Design review of the part built by this model. Coordinates are the model's own, in mm. Face numbers are marked on the shaded views. A direction names the side the tool comes from. Give positions to 0.01 mm unless a question says otherwise; leave off trailing zeros. Loops run counter-clockwise (first coordinate to the right, second up) from the corner with the lowest first, then second, coordinate; pieces in that order, holes last. Notation, with made-up numbers: (23, 75.25) -> (39, 75.25) arc R18 ccw to (39, 90.25) -> close; hole circle Ø9 at (47, -38). An arc over 180 degrees is marked (long way). Answer in a Markdown table with one row per item. Add a question column.
(1) For line 1 (Z direction, x = 7.5, y = -46.5); line 2 (Z direction, x = 11.5, y = 6.5); line 3 (Y direction, x = 7.5, z = -3.5), list the stretches that pass through material, from the lowest coordinate up.
(2) For pin 1 (6.5 mm diameter, centred on x = 7.5, z = 15, fed in from +Y); pin 2 (6 mm diameter, centred on x = 11, y = -3.5, fed in from -Z); pin 3 (5 mm diameter, centred on x = 7.5, y = 8.48, fed in from +Z); pin 4 (3 mm diameter, centred on x = 7.5, z = -15, fed in from +Y), all flat-tipped, find the tip position at first contact; note any pin that passes through.
(3) Consider section D-D on x = 3.25. Write out the cut boundary in (y, z).
(4) Draft analysis for pull direction Y (two halves, no side actions). For the marked faces 4, 5 and 6, state which applies: +Y half, -Y half, draft (parallel to the pull), parting line (faces both ways), or undercut.
(5) Consider section A-A on y = 0. Write out the cut boundary in (x, z).
(6) For the marked faces 1, 2 and 3, list the 3-axis set-ups (+Z, -Z, +X, -X, +Y, -Y) from which the entire face can be reached by the end or side of a thin tool; tool diameter is ignored.
(7) Consider section C-C on z = -15. Write out the cut boundary in (x, y).
(8) Consider section B-B on x = 7.5. Write out the cut boundary in (y, z).
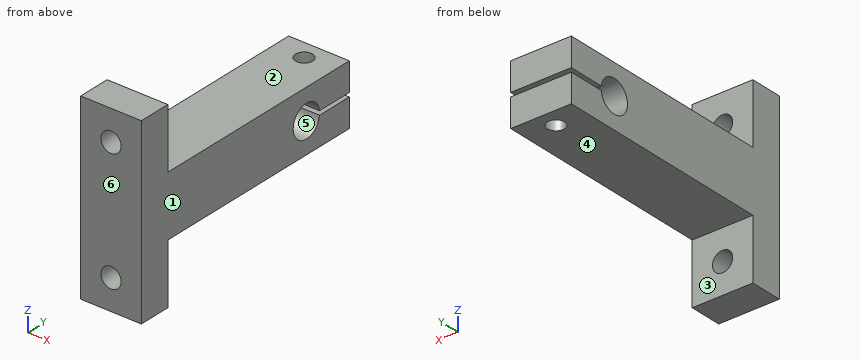
Autodesk Inventor part; units mm, degrees
ref_plane "YZ Plane" through (0, 0, 0) normal (1, 0, 0) x (0, 1, 0)
ref_plane "XZ Plane" through (0, 0, 0) normal (0, 1, 0) x (-1, 0, 0)
ref_plane "XY Plane" through (0, 0, 0) normal (0, 0, 1) x (1, 0, 0)
sketch "Sketch1" plane through (0, 0, 0) normal (1, 0, 0) x (0, 1, 0)
  line L0 (-50, 22.5) -> (-50, -22.5)
  line L1 (-50, -22.5) -> (-42, -22.5)
  line L2 (-42, -22.5) -> (-42, -7.5)
  line L3 (-42, -7.5) -> (13, -7.5)
  line L4 (13, -7.5) -> (13, -0.5)
  line L5 (-50, 22.5) -> (-42, 22.5)
  line L6 (-42, 22.5) -> (-42, 7.5)
  line L7 (-42, 7.5) -> (13, 7.5)
  line L8 (13, 7.5) -> (13, 0.5)
  circle A0 centre (0, 0) radius 4
  line L9 (13, 0.5) -> (0, 0.5)
  line L10 (0, 0.5) -> (0, -0.5)
  line L11 (0, -0.5) -> (13, -0.5)
  line L12 (0, 0) -> (-35.797, 0) construction
  dimension "d0" = 8
  dimension "d1" = 1
  dimension "d2" = 7
  dimension "d3" = 15
  dimension "d5" = 55
  dimension "d6" = 8
  dimension "d11" = 50
extrude "Extrusion1" add sketch "Sketch1" along normal blind 15 contours L5 L6 L7 L8 L9 A0 L11 L4 L3 L2 L1 L0 | L9 L10 L11 A0 picked at (-1.3236, -0.1605)
extrude "Extrusion2" cut sketch "Sketch1" along normal through all contours L9 L10 L11 A0 | A0 L11 L10 L9
sketch "Sketch2" plane through (0, -42, 22.5) normal (0, 1, 0) x (1, 0, 0)
  circle A0 centre (7.5, 7.5) radius 2.5
  circle A1 centre (7.5, 37.5) radius 2.5
  line L0 (0, 45) -> (0, 30)
  line L1 (0, 15) -> (0, 0)
  line L2 (0, 45) -> (0, 30)
  line L3 (0, 30) -> (15, 30)
  line L4 (15, 45) -> (15, 30)
  line L5 (0, 45) -> (15, 45)
  line L6 (0, 15) -> (0, 0)
  line L7 (0, 0) -> (15, 0)
  line L8 (15, 15) -> (15, 0)
  line L9 (0, 15) -> (15, 15)
  line L10 (7.5, 7.5) -> (0, 7.5)
  line L11 (0, 0) -> (0, 45)
  line L12 (7.5, 37.5) -> (15, 37.5)
  line L13 (15, 0) -> (15, 45)
  line L14 (7.5, 37.5) -> (0, 37.5)
  line L15 (7.5, 37.5) -> (7.5, 30)
  line L16 (7.5, 37.5) -> (7.5, 45)
  line L17 (0, 45) -> (15, 45)
  line L18 (7.5, 7.5) -> (15, 7.5)
  line L19 (7.5, 7.5) -> (7.5, 15)
  line L20 (0, 15) -> (15, 15)
  line L21 (7.5, 7.5) -> (7.5, 0)
  line L22 (0, 0) -> (15, 0)
  point P0 (0, 22.5)
  dimension "d12" = 5
extrude "Extrusion3" cut sketch "Sketch2" against normal through all contours L18 L19 A0 | A0 L21 L18 | L19 L10 A0 | A0 L10 L21 | L15 L12 A1 | A1 L14 L15 | L12 L16 A1 | A1 L16 L14
sketch "Sketch3" plane through (0, -42, 7.5) normal (0, 0, 1) x (1, 0, 0)
  circle A0 centre (7.5, 50.4843) radius 2.125
  line L0 (7.5, 50.4843) -> (0, 50.4843) construction
  line L1 (7.5, 50.4843) -> (15, 50.4843) construction
  line L2 (0, 55) -> (0, 0)
  line L3 (0, 55) -> (15, 55)
  line L4 (15, 45.9686) -> (15, 55)
  line L5 (15, 55) -> (15, 0)
  line L6 (7.5, 50.4843) -> (15, 55) construction
  line L7 (15, 45.9686) -> (15, 38)
  line L8 (15, 45.9686) -> (7.5, 50.4843) construction
  point P0 (0, 42)
  point P1 (15, 42)
  dimension "d15" = 4.25
extrude "Extrusion4" cut sketch "Sketch3" against normal through all
properties part number "XRodClamp"
Values follow:
| question | item | result |
|---|---|---|
| 1 | line 1 | -22.5 to -17.5, -12.5 to 12.5, 17.5 to 22.5 |
| 1 | line 2 | -7.5 to -0.5, 0.5 to 7.5 |
| 1 | line 3 | -50 to -1.94, 1.94 to 6.36, 10.61 to 13 |
| 2 | pin 1 | y = -42 |
| 2 | pin 2 | z = -7.5 |
| 2 | pin 3 | z = 7.5 |
| 2 | pin 4 | through |
| 3 | outline | (-50, -22.5) -> (-42, -22.5) -> (-42, -7.5) -> (13, -7.5) -> (13, -0.5) -> (3.97, -0.5) arc R4 cw (long way) to (3.97, 0.5) -> (13, 0.5) -> (13, 7.5) -> (-42, 7.5) -> (-42, 22.5) -> (-50, 22.5) -> close |
| 4 | face 4 | draft |
| 4 | face 5 | undercut |
| 4 | face 6 | -Y half |
| 5 | outline | (0, -7.5) -> (15, -7.5) -> (15, -4) -> (0, -4) -> close; (0, 4) -> (15, 4) -> (15, 7.5) -> (0, 7.5) -> close |
| 6 | face 1 | +Z, -Z, +X, +Y, -Y |
| 6 | face 2 | +Z, +X, -X, +Y |
| 6 | face 3 | -Z, +X, -X, +Y |
| 7 | outline | (0, -50) -> (5, -50) -> (5, -42) -> (0, -42) -> close; (10, -50) -> (15, -50) -> (15, -42) -> (10, -42) -> close |
| 8 | outline | (-50, -22.5) -> (-42, -22.5) -> (-42, -17.5) -> (-50, -17.5) -> close; (-50, -12.5) -> (-42, -12.5) -> (-42, -7.5) -> (6.36, -7.5) -> (6.36, -0.5) -> (3.97, -0.5) arc R4 cw (long way) to (3.97, 0.5) -> (6.36, 0.5) -> (6.36, 7.5) -> (-42, 7.5) -> (-42, 12.5) -> (-50, 12.5) -> close; (-50, 17.5) -> (-42, 17.5) -> (-42, 22.5) -> (-50, 22.5) -> close; (10.61, -7.5) -> (13, -7.5) -> (13, -0.5) -> (10.61, -0.5) -> close; (10.61, 0.5) -> (13, 0.5) -> (13, 7.5) -> (10.61, 7.5) -> close |
